The listing builds one solid part. Answer for the finished solid, in the listing's coordinates (mm). Give positions to 0.01 mm unless a question says otherwise; leave off trailing zeros. Order: outer loops, then holes, each group sorted by start corner. A loop starts at its lowest first (then second) coordinate and runs counter-clockwise, first axis right, second up.
```python
from build123d import *

# Parameters (mm, degrees)
SKETCH1_W           = 30
SKETCH1_H           = 30
BOSS_EXTRUDE1_DEPTH = 10
SKETCH3_R           = 13.75
SKETCH3_R_2         = 2
CUT_EXTRUDE1_DEPTH  = 10
FILLET1_R           = 2


with BuildPart() as part:
    # Sketch1 → Boss-Extrude1 (new body)
    with BuildSketch(Plane.XY):
        with Locations((15, 15)):
            Rectangle(SKETCH1_W, SKETCH1_H)
    extrude(amount=BOSS_EXTRUDE1_DEPTH)

    # Sketch3 → Cut-Extrude1 (cut)
    with BuildSketch(Plane.XY.offset(10)):
        with Locations((15, 15)):
            Circle(SKETCH3_R)
        with Locations((3, 27)):
            Circle(SKETCH3_R_2)
        with Locations((3, 3)):
            Circle(SKETCH3_R_2)
        with Locations((27, 3)):
            Circle(SKETCH3_R_2)
        with Locations((27, 27)):
            Circle(SKETCH3_R_2)
    extrude(amount=-CUT_EXTRUDE1_DEPTH, mode=Mode.SUBTRACT)

    # Fillet1
    fillet1_edges = [part.edges().sort_by_distance(p)[0] for p in [
        (0, 30, 5),
        (30, 30, 5),
        (30, 0, 5),
        (0, 0, 5),
    ]]
    fillet(fillet1_edges, radius=FILLET1_R)


solid = part.part
```
1) Straight lines are drawn through the part: probe 1 along Y at (x, z) = (15, 2.5); probe 2 along Y at (x, z) = (2.5, 6.75); probe 3 along Y at (x, z) = (27, 6.25). For each, find the intervals that lie inside material, in ascending order.
Geometry says:
probe 1: y = 0 to 1.25, 28.75 to 30
probe 2: y = 0 to 1.06, 4.94 to 9.27, 20.73 to 25.06, 28.94 to 30
probe 3: y = 0 to 1, 5 to 8.29, 21.71 to 25, 29 to 30
2) Find section D-D (y = 3). Write down the section's boundary in (x, z).
Geometry says:
outline: (0, 0) - (1, 0) - (1, 10) - (0, 10) - close; (5, 0) - (8.29, 0) - (8.29, 10) - (5, 10) - close; (21.71, 0) - (25, 0) - (25, 10) - (21.71, 10) - close; (29, 0) - (30, 0) - (30, 10) - (29, 10) - close
3) Find section B-B (x = 15). Write down the section's boundary in (y, z), then the cut area to 3 significant figures.
Geometry says:
outline: (0, 0) - (1.25, 0) - (1.25, 10) - (0, 10) - close; (28.75, 0) - (30, 0) - (30, 10) - (28.75, 10) - close
area: 25.0 mm2
4) For a pull along Y with two mould halves and no side action, classify faces 1 (the cylindrical face through (4.866, 24.293, 5.07)), 2 (the flat face through (8.3, 2.8, 10)), 3 (the cylindrical face through (27.923, 25.226, 5.07)), 4 (the cylindrical face through (29.4, 0.57, 5.07)) as +Y half, -Y half, draft (parallel to the pull), parting line (faces both ways), or undercut.
Geometry says:
face 1: undercut
face 2: draft
face 3: undercut
face 4: -Y half
5) Find section A-A (z = 4). Write down the section's boundary in (x, y), then the cut area to 3 significant figures.
Geometry says:
outline: (0, 2) arc R2 ccw to (2, 0) - (28, 0) arc R2 ccw to (30, 2) - (30, 28) arc R2 ccw to (28, 30) - (2, 30) arc R2 ccw to (0, 28) - close; hole circle Ø4 at (3, 3); hole circle Ø4 at (3, 27); hole circle Ø27.5 at (15, 15); hole circle Ø4 at (27, 3); hole circle Ø4 at (27, 27)
area: 252 mm2
6) Given P1, Ø5, axis at x = 24.5, y = 17, coming from the -Z side, flat-ended and moving along its own axis, determine where the tip first touches the part or whether it passes through.
Geometry says:
P1: passes through
